Geometry check sheet. Reference: the model listing, model coordinates, mm. Give positions to 0.01 mm unless a question says otherwise; leave off trailing zeros. Loops run counter-clockwise (first coordinate to the right, second up) from the corner with the lowest first, then second, coordinate; pieces in that order, holes last. Notation, with made-up numbers: (8, 33.5) -> (23, 33.5) arc R16 cw to (23, 49.5) -> close; hole circle Ø4 at (-1, 52.5). An arc over 180 degrees is marked (long way). Answer as a JSON object with one key per item and string values.
from build123d import *

# Parameters (mm, degrees)
SKETCH_1_R          = 1.5
EXTRUDE_1_DEPTH     = 2.5
SKETCH_2_W          = 21.5
SKETCH_2_H          = 6.25
CUT_EXTRUDE_1_DEPTH = 3.5000001
SKETCH_3_R          = 10
CUT_EXTRUDE_2_DEPTH = 3.5000001


with BuildPart() as part:
    # 草图1 → 凸台-拉伸1 (new body)
    with BuildSketch(Plane(origin=(0, 0, 0), x_dir=(1, 0, 0), z_dir=(0, 1, 0))):
        with BuildLine():
            Line((-128.499999999, -16), (-128.499999999, 16))
            add(Edge.make_bspline(
                [(-93.499999999, 75.000000013), (-111.61760277, 74.009879458), (-123.133759969, 57.24109691), (-128.499999999, 30.447414919), (-128.499999999, 16)],
                knots=[0, 0, 0, 0, 0.426208918, 0.752892545, 0.752892545, 0.752892545, 0.752892545], degree=3))
            Line((-93.499999999, 75.000000013), (-93.499999999, 50))
            Line((-93.499999999, 50), (-17.5, 50))
            Line((-17.5, 50), (-17.5, 75.000000013))
            Line((-17.5, 75.000000013), (17.5, 75.000000013))
            Line((17.5, 75.000000013), (17.5, 50))
            Line((17.5, 50), (93.499999999, 50))
            Line((93.499999999, 50), (93.499999999, 75.000000013))
            add(Edge.make_bspline(
                [(93.499999999, 75.000000013), (111.61760277, 74.009879458), (123.133759969, 57.24109691), (128.499999999, 30.447414919), (128.499999999, 16)],
                knots=[0, 0, 0, 0, 0.426208918, 0.752892545, 0.752892545, 0.752892545, 0.752892545], degree=3))
            Line((128.499999999, 16), (128.499999999, -16))
            add(Edge.make_bspline(
                [(93.499999999, -75.000000013), (111.61760277, -74.009879458), (123.133759969, -57.24109691), (128.499999999, -30.447414919), (128.499999999, -16)],
                knots=[0, 0, 0, 0, 0.426208918, 0.752892545, 0.752892545, 0.752892545, 0.752892545], degree=3))
            Line((93.499999999, -75.000000013), (93.499999999, -50))
            Line((93.499999999, -50), (17.5, -50))
            Line((17.5, -50), (17.5, -75.000000013))
            Line((17.5, -75.000000013), (-17.5, -75.000000013))
            Line((-17.5, -75.000000013), (-17.5, -50))
            Line((-17.5, -50), (-93.499999999, -50))
            Line((-93.499999999, -50), (-93.499999999, -75.000000013))
            add(Edge.make_bspline(
                [(-93.499999999, -75.000000013), (-111.61760277, -74.009879458), (-123.133759969, -57.24109691), (-128.499999999, -30.447414919), (-128.499999999, -16)],
                knots=[0, 0, 0, 0, 0.426208918, 0.752892545, 0.752892545, 0.752892545, 0.752892545], degree=3))
        make_face()
        with Locations((-108.499999999, 60)):
            Circle(SKETCH_1_R, mode=Mode.SUBTRACT)
        with Locations((-108.499999999, -60)):
            Circle(SKETCH_1_R, mode=Mode.SUBTRACT)
        with Locations((108.499999999, -60)):
            Circle(SKETCH_1_R, mode=Mode.SUBTRACT)
        with Locations((108.499999999, 60)):
            Circle(SKETCH_1_R, mode=Mode.SUBTRACT)
        with Locations((7, 70.000000013)):
            Circle(SKETCH_1_R, mode=Mode.SUBTRACT)
        with Locations((-7, 70.000000013)):
            Circle(SKETCH_1_R, mode=Mode.SUBTRACT)
        with Locations((7, -70.000000013)):
            Circle(SKETCH_1_R, mode=Mode.SUBTRACT)
        with Locations((-7, -70.000000013)):
            Circle(SKETCH_1_R, mode=Mode.SUBTRACT)
    extrude(amount=EXTRUDE_1_DEPTH)

    # 草图2 → 切除-拉伸1 (cut, through all)
    with BuildSketch(Plane(origin=(0, 2.5, 0), x_dir=(1, 0, 0), z_dir=(0, 1, 0))):
        with Locations((57.25, 21.875)):
            Rectangle(SKETCH_2_W, SKETCH_2_H)
        with Locations((57.25, -21.875)):
            Rectangle(SKETCH_2_W, SKETCH_2_H)
    extrude(amount=-CUT_EXTRUDE_1_DEPTH, mode=Mode.SUBTRACT)

    # 草图3 → 切除-拉伸2 (cut, through all)
    with BuildSketch(Plane(origin=(0, 2.5, 0), x_dir=(1, 0, 0), z_dir=(0, 1, 0))):
        with Locations((97.499999999, 0)):
            Circle(SKETCH_3_R)
    extrude(amount=-CUT_EXTRUDE_2_DEPTH, mode=Mode.SUBTRACT)


solid = part.part
1) Material ranges on line 1 along Z through (x, y) = (7, 1.75); line 2 along X through (y, z) = (0.95, 60); line 3 along X through (y, z) = (1, -64.5), recorded low to high. Write a range as from..to.
Geometry check:
{"line 1": "z = -75..-71.5, -68.5..68.5, 71.5..75", "line 2": "x = -119.12..-110, -107..-93.5, -17.5..17.5, 93.5..107, 110..119.12", "line 3": "x = -116.21..-93.5, -17.5..17.5, 93.5..116.21"}
2) Draft check along Z on faces 1 (the face through (107.04, 1.27, -3)), 2 (the face through (2, 2.5, -1)). Enter one of: pulls with the +Z half, pulls with the -Z half, needs draft (parallel to the pull), parting line crosses it, or undercut.
Geometry check:
{"face 1": "undercut", "face 2": "needs draft"}
3) Section check C-C on x = -45. Record the cut outline in (y, z), plus the area to 3 significant figures.
Geometry check:
{"outline": "(0, -50) -> (2.5, -50) -> (2.5, 50) -> (0, 50) -> close", "area": "250 mm2"}
4) Section check A-A on z = 0. Record the cut outline in (x, y).
Geometry check:
{"outline": "(-128.5, 0) -> (87.5, 0) -> (87.5, 2.5) -> (-128.5, 2.5) -> close; (107.5, 0) -> (128.5, 0) -> (128.5, 2.5) -> (107.5, 2.5) -> close"}
5) Section check B-B on y = 1.4. Count the separate pieces of the cut face and the enclosed holes in it, plus the area to 3 significant figures.
Geometry check:
{"separate pieces": "1", "enclosed holes": "11", "area": "28,800 mm2"}
6) Depth check by flat-ended pin: P1, Ø1.2, axis at x = 55.5, y = 1, coming from the -Z side; P2, Ø1.2, axis at x = 62, y = 1.5, coming from the +Z side; P3, Ø1.2, axis at y = 1.5, z = -62, coming from the -X side. Enter the tip coordinate at first touch or a pass-through.
Geometry check:
{"P1": "stops at z = -50", "P2": "stops at z = 50", "P3": "stops at x = -118.32"}
